from build123d import *

# Parameters (mm, degrees)
SALIENTE_EXTRUIR1_DEPTH = 1.4


with BuildPart() as part:
    # Croquis1 → Saliente-Extruir1 (new body)
    with BuildSketch(Plane.XY):
        with BuildLine():
            Line((2.6, 4), (-2, 4))
            ThreePointArc((-2, 4), (-3.414213562, 3.414213562), (-4, 2))
            Line((-4, 2), (-4, -2.6))
            Line((-4, -2.6), (-2.756314656, -2.6))
            ThreePointArc((-2.756314656, -2.6), (-2.259416606, -2.293841943), (-2.309436887, -1.712345253))
            ThreePointArc((-2.309436887, -1.712345253), (-2.032931996, 2.032931996), (1.712345253, 2.309436887))
            ThreePointArc((1.712345253, 2.309436887), (2.293841943, 2.259416606), (2.6, 2.756314656))
            Line((2.6, 2.756314656), (2.6, 4))
        make_face()
    extrude(amount=SALIENTE_EXTRUIR1_DEPTH)


solid = part.part
Could you check a few things on this model? Use its own coordinates, in mm. Give positions to 0.01 mm unless a question says otherwise; leave off trailing zeros. Order: outer loops, then holes, each group sorted by start corner. A loop starts at its lowest first (then second) coordinate and runs counter-clockwise, first axis right, second up. Notation, with made-up numbers: (70.25, 63) - (121.25, 63) arc R24 cw to (121.25, 74) - close; hole circle Ø1 at (26.5, 27). An arc over 180 degrees is marked (long way). One line per item, written item: value. Start each with the question number.
1. Imagine slicing it at D-D on x = -0.25. List the corners of the cut face in (y, z) for me.
2. If I drill on probe 1 along Y at (x, z) = (2, 0.7); probe 2 along Y at (x, z) = (-2.5, 1); probe 3 along Y at (x, z) = (-1.5, 0.2), over which ranges is the centre line in solid material (lowest first)?
3. Imagine slicing it at C-C on y = -1.25. List the corners of the cut face in (x, z) for me, plus the area to 3 significant figures.
4. Thinking about a two-plate mould opening in X: for faces 1 (the face through (2.286, 2.256, 0.69)), 2 (the face through (-2.2, 2.2, 1.4)), 3 (the face through (-2.263, -2.301, 0.69)), which applies, +X half, -X half, draft (parallel to the pull), parting line (faces both ways), or undercut?
5. Imagine slicing it at A-A on x = -2.5. List the corners of the cut face in (y, z) for me, plus the area to 3 significant figures.
6. Imagine slicing it at B-B on z = 0.4. List the corners of the cut face in (x, y) for me (3 decimals).
Values:
1. outline: (2.86, 0) - (4, 0) - (4, 1.4) - (2.86, 1.4) - close
2. probe 1: 2.2 to 4
2. probe 2: -2.54 to -1.42, 1.42 to 3.94
2. probe 3: 2.45 to 4
3. outline: (-4, 0) - (-2.59, 0) - (-2.59, 1.4) - (-4, 1.4) - close
3. area: 1.98 mm²
4. face 1: undercut
4. face 2: draft
4. face 3: +X half
5. outline: (-2.54, 0) - (-1.42, 0) - (-1.42, 1.4) - (-2.54, 1.4) - close; (1.42, 0) - (3.94, 0) - (3.94, 1.4) - (1.42, 1.4) - close
5. area: 5.09 mm²
6. outline: (-4, -2.6) - (-2.756, -2.6) arc R0.556 ccw to (-2.309, -1.712) arc R2.875 cw to (1.712, 2.309) arc R0.556 ccw to (2.6, 2.756) - (2.6, 4) - (-2, 4) arc R2 ccw to (-4, 2) - close
